```python
from build123d import *

# Parameters (mm, degrees)
F0_W     = 61.8317574263
F0_H     = 44.1648438573
F1_DEPTH = 8.5
F2_R     = 2
F4_DEPTH = 56
F5_R     = 2.5
F6_DEPTH = 25
F6_TAPER = -45


with BuildPart() as f1:
    # F0 (on Top) → F1 (new body)
    with BuildSketch(Plane.XY):
        with Locations((3.5895518959, 0)):
            Rectangle(F0_W, F0_H)
    extrude(amount=F1_DEPTH)

    # F2
    f2_edges = [f1.edges().sort_by_distance(p)[0] for p in [
        (-27.326327, -22.082422, 4.25),
        (34.505431, -22.082422, 4.25),
        (-27.326327, 22.082422, 4.25),
        (34.505431, 22.082422, 4.25),
    ]]
    fillet(f2_edges, radius=F2_R)

    # F3 (on face) → F4 (cut)
    with BuildSketch(Plane(origin=(-27.3263268173, 0, 0), x_dir=(0, -1, 0), z_dir=(-1, 0, 0))):
        with BuildLine():
            ThreePointArc((-18.1670283088, 3), (-17.87413509, 2.2928932188), (-17.1670283088, 2))
            Line((-17.1670283088, 2), (17.1670283088, 2))
            ThreePointArc((17.1670283088, 2), (17.87413509, 2.2928932188), (18.1670283088, 3))
            Line((18.1670283088, 3), (18.1670283088, 6.3671339807))
            Line((18.1670283088, 6.3671339807), (15.3303788975, 6.3671339807))
            Line((15.3303788975, 6.3671339807), (15.3303788975, 8.5))
            Line((15.3303788975, 8.5), (-15.4332136735, 8.5))
            Line((-15.4332136735, 8.5), (-15.4332136735, 6.3671339807))
            Line((-15.4332136735, 6.3671339807), (-18.1670283088, 6.3671339807))
            Line((-18.1670283088, 6.3671339807), (-18.1670283088, 3))
        make_face()
    extrude(amount=-F4_DEPTH, mode=Mode.SUBTRACT)

    # F5 (on Top) → F6 (cut)
    with BuildSketch(Plane.XY):
        Circle(F5_R)
    extrude(amount=F6_DEPTH, taper=F6_TAPER, mode=Mode.SUBTRACT)


solid = f1.part
```
Input: part model. Units: mm. Frame: model coordinates. A direction names the side the tool comes from. Coordinates: 2 decimals unless noted, no trailing zeros. Loops run counter-clockwise (first coordinate to the right, second up) from the corner with the lowest first, then second, coordinate; pieces in that order, holes last. Notation, with made-up numbers: (29.25, -35) - (44.25, -35) arc R31 cw to (44.25, 4) - close; hole circle Ø10 at (27.5, -26.5). An arc over 180 degrees is marked (long way). Answer in a Markdown table with one row per item.
(1) Material intervals for L1, parallel to Y at x = -5, z = 7; L2, parallel to Y at x = 25.5, z = 5.25; L3, parallel to X at y = 12, z = 2.5, sorted ascending. Write a range as from..to.
Model answer:
| item | result |
|---|---|
| L1 | y = -22.08..-15.33, 15.43..22.08 |
| L2 | y = -22.08..-18.17, 18.17..22.08 |
| L3 | x = 28.67..34.51 |
(2) Mould query, pull axis Y, two halves, no side actions, for faces 1 (the face through (-27.326, -0.1, 1.7)), 2 (the face through (33.904, -21.512, 4.31)), 3 (the face through (0, -18.167, 5)). Classes: pulls with the +Y half, pulls with the -Y half, needs draft (parallel to the pull), parting line crosses it, or undercut.
Model answer:
| item | result |
|---|---|
| face 1 | needs draft |
| face 2 | pulls with the -Y half |
| face 3 | undercut |
(3) Set-up query: faces 4 (the face through (0, -15.33, 7)), 5 (the face through (3, -22.082, 4)), 6 (the face through (0, -17, 6.367)). Return all of +Z, -Z, +X, -X, +Y, -Y with unobstructed straight access to the full face (end or side cutting, diameter ignored); none if empty.
Model answer:
| item | result |
|---|---|
| face 4 | +Z, -X |
| face 5 | +Z, -Z, +X, -X, -Y |
| face 6 | -X |
(4) Pin query (flat end, axial travel): P1, Ø6, axis at x = 21.5, y = -11, coming from the +Z side; P2, Ø2, axis at y = 3.5, z = 4.5, coming from the -X side. Return the tip coordinate at first contact, or that it passes through.
Model answer:
| item | result |
|---|---|
| P1 | stops at z = 2 |
| P2 | stops at x = 28.67 |
(5) Cut plane D-D on y = -11.5. Output: boundary loops of the cut face in (x, z).
Model answer:
| item | result |
|---|---|
| outline | (-27.33, 0) - (34.51, 0) - (34.51, 8.5) - (28.67, 8.5) - (28.67, 2) - (-27.33, 2) - close |
(6) Cut plane A-A on x = 0. Output: boundary loops of the cut face in (y, z).
Model answer:
| item | result |
|---|---|
| outline | (-22.08, 0) - (-2.5, 0) - (-4.5, 2) - (-17.17, 2) arc R1 cw to (-18.17, 3) - (-18.17, 6.37) - (-15.33, 6.37) - (-15.33, 8.5) - (-22.08, 8.5) - close; (2.5, 0) - (22.08, 0) - (22.08, 8.5) - (15.43, 8.5) - (15.43, 6.37) - (18.17, 6.37) - (18.17, 3) arc R1 cw to (17.17, 2) - (4.5, 2) - close |
(7) Cut plane C-C on x = 16.5. Output: boundary loops of the cut face in (y, z), plus the area to 3 significant figures.
Model answer:
| item | result |
|---|---|
| outline | (-22.08, 0) - (22.08, 0) - (22.08, 8.5) - (15.43, 8.5) - (15.43, 6.37) - (18.17, 6.37) - (18.17, 3) arc R1 cw to (17.17, 2) - (-17.17, 2) arc R1 cw to (-18.17, 3) - (-18.17, 6.37) - (-15.33, 6.37) - (-15.33, 8.5) - (-22.08, 8.5) - close |
| area | 152 mm² |
(8) Cut plane B-B on y = 16.5. Output: boundary loops of the cut face in (x, z).
Model answer:
| item | result |
|---|---|
| outline | (-27.33, 0) - (34.51, 0) - (34.51, 8.5) - (-27.33, 8.5) - (-27.33, 6.37) - (28.67, 6.37) - (28.67, 2) - (-27.33, 2) - close |
